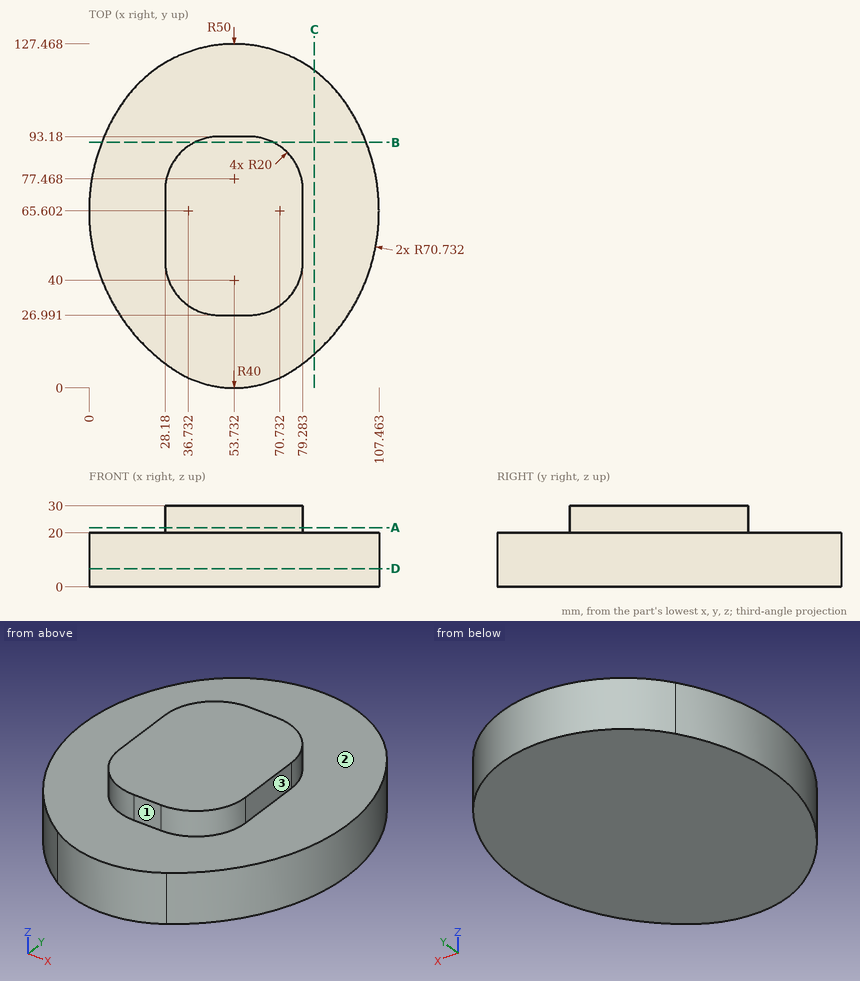
Answer from the drawing. Dimensions are ordinates in mm from the lowest x, y and z of the part. A direction names the side the tool comes from. Coordinates: 2 decimals unless noted, no trailing zeros. Write each loop counter-clockwise with the first axis right and the second up, starting at its lowest first coordinate (ties: lowest second). Pieces come first, ordered by that corner, then holes. Notation, with made-up numbers: M 53,0 L 58,0 A27 ccw 58,20 Z; hole C -38,78 d7. An arc over 180 degrees is marked long. Put each result on its own line as item: value. Start each with the question number.
1. A cutting plane is placed at C-C on x = 83.5. Write down the section's boundary in (y, z).
2. A cutting plane is placed at B-B on y = 91. Write down the section's boundary in (x, z).
3. A cutting plane is placed at D-D on z = 6.75. Write down the section's boundary in (x, y) (1 decimal).
4. A cutting plane is placed at A-A on z = 22. Write down the section's boundary in (x, y).
5. Consider line 1 (Z direction, x = 9, y = 34); line 2 (X direction, y = 79.5, z = 4.75) (1 decimal); line 3 (Y direction, x = 68, z = 20.75). Determine where each line is inside the solid, lowest interval first. Write a range as from..to.
6. Flat-ended cylindrical pins translate along their axes: P1, Ø3, axis at x = 35.5, y = 16, coming from the +Z side; P2, Ø8, axis at x = 89.5, z = 22, coming from the -Y side (1 decimal); P3, Ø11, axis at y = 59.5, z = 23, coming from the -X side. Find the tip coordinate at first contact, or state that the pin passes through.
7. Which of the six approach directions +Z, -Z, +X, -X, +Y, -Y give full straight-line access (tool end or side, diameter ignored) to the marked faces 1, 2 and 3?
Resolved:
1. outline: M 12.54,0 L 117.64,0 L 117.64,20 L 12.54,20 Z
2. outline: M 4.72,0 L 102.75,0 L 102.75,20 L 68.36,20 L 68.36,30 L 39.1,30 L 39.1,20 L 4.72,20 Z
3. outline: M 12.7,106.1 A70.7 ccw 31.6,6.7 A40 ccw 75.9,6.7 A70.7 ccw 94.7,106.1 A50 ccw Z
4. outline: M 28.18,46.99 A20 ccw 48.18,26.99 L 59.28,26.99 A20 ccw 79.28,46.99 L 79.28,73.18 A20 ccw 59.28,93.18 L 48.18,93.18 A20 ccw 28.18,73.18 Z
5. line 1: z = 0..20
5. line 2: x = 1.4..106.1
5. line 3: y = 28.99..91.18
6. P1: stops at z = 20
6. P2: stops at y = 14.9
6. P3: stops at x = 0.02
7. face 1: +Z, +X, -X, -Y
7. face 2: +Z
7. face 3: +Z, +X, +Y, -Y
